Check sheet for the modelled part. Datum: model origin and axes. Units: mm. Coordinates: 2 decimals unless noted, no trailing zeros. Loops run counter-clockwise (first coordinate to the right, second up) from the corner with the lowest first, then second, coordinate; pieces in that order, holes last. Notation, with made-up numbers: M -3,62.5 L 55,62.5 A12 cw 55,77.5 Z; hole C -22,59 d4. An arc over 180 degrees is marked long. Answer as CSV lines item,"result". Start each with the question number.
Autodesk Inventor part; units mm, degrees
ref_plane "Work Plane1" through (0, 0, 20) normal (1, 0, 0) x (0, 0, -1)
ref_plane "Work Plane2" through (-25, 0, 0) normal (0, 0, 1) x (1, 0, 0)
ref_plane "YZ Plane" through (0, 0, 0) normal (1, 0, 0) x (0, 1, 0)
sketch "Sketch1" plane through (0, 0, 0) normal (0, 1, 0) x (-1, 0, 0)
  circle A0 centre (0, 0) radius 6.5
  line L0 (25, 20) -> (-25, 20)
  line L1 (-25, 20) -> (-25, -20)
  line L2 (-25, -20) -> (25, -20)
  line L3 (25, -20) -> (25, 20)
  line L4 (25, 20) -> (-25, -20) construction
  line L5 (-25, 20) -> (25, -20) construction
  line L6 (-25, 0) -> (-30, 0)
  line L7 (-30, 0) -> (-30, -10)
  line L8 (-30, -10) -> (-25, -10)
  line L9 (-25, -10) -> (-25, 0)
  line L10 (-30, 0) -> (-25, 0)
  line L11 (-25, 0) -> (-25, 10)
  line L12 (-25, 10) -> (-30, 10)
  line L13 (-30, 10) -> (-30, 0)
  line L14 (-25, 10) -> (-25, 5)
  line L15 (-25, 5) -> (-26.5, 5)
  line L16 (-26.5, 5) -> (-28, 5)
  line L17 (-28, 5) -> (-28, -5)
  line L18 (-28, -5) -> (-26.5, -5)
  line L19 (-26.5, -5) -> (-26.5, 5)
  line L20 (0, 0) -> (0, -20)
  line L21 (30, 0) -> (30, -10)
  line L22 (30, -10) -> (25, -10)
  line L23 (26.5, -5) -> (26.5, 5)
  line L24 (28, 5) -> (28, -5)
  line L25 (28, -5) -> (26.5, -5)
  line L26 (26.5, 5) -> (28, 5)
  line L27 (25, 10) -> (30, 10)
  line L28 (30, 10) -> (30, 0)
  dimension "d0" = 13
  dimension "d1" = 50
  dimension "d2" = 40
  dimension "d3" = 5
  dimension "d4" = 10
  dimension "d5" = 5
  dimension "d6" = 10
  dimension "d7" = 5
  dimension "d8" = 1.5
  dimension "d9" = 1.5
  dimension "d10" = 10
extrude "Extrusion1" add sketch "Sketch1" along normal blind 1.5 contours L2 L1 L0 L3 | L8 L7 L6 L17 L18 L19 L1 | L3 L27 L28 L21 L22 | L6 L19 L15 L1 | L15 L16 L17 L6 L13 L12 L1
sketch "Sketch2" plane through (0, 1.5, 0) normal (0, 1, 0) x (1, 0, 0)
  line L0 (0, 0) -> (22.5, 0)
  line L1 (22.5, 0) -> (22.5, 17.5)
  line L2 (25, 20) -> (-25, 20)
  circle A0 centre (22.5, 17.5) radius 1.5
  dimension "d13" = 22.5
  dimension "d14" = 17.5
  dimension "d15" = 3
extrude "Extrusion2" cut sketch "Sketch2" against normal blind 1.5
ref_plane "Work Plane1" through (0, 0, 20) normal (1, 0, 0) x (0, 0, -1)
ref_plane "Work Plane2" through (-25, 0, 0) normal (0, 0, 1) x (1, 0, 0)
mirror "Mirror1" about plane through (0, 0, 20) normal (1, 0, 0) of "Extrusion2"
mirror "Mirror2" about plane through (-25, 0, 0) normal (0, 0, 1) of "Extrusion2", "Mirror1"
sketch "Sketch3" plane through (0, 1.5, 0) normal (0, 1, 0) x (1, 0, 0)
  line L0 (25, 10) -> (25, 20)
  line L1 (25, 20) -> (20, 20)
  line L2 (25, 20) -> (-25, 20)
  line L3 (0, 0) -> (0, 9)
  line L4 (20, 20) -> (9.6256, 9) construction
  line L5 (9.6256, 9) -> (0, 9) construction
  spline S0 degree 2 poles (20, 20) (9.6256, 9) (0, 9) knots 1 1 1 2 2 2
  line L6 (0, 0) -> (9.6256, 0)
  line L7 (-20, 20) -> (-9.6256, 9) construction
  line L8 (-9.6256, 9) -> (0, 9) construction
  spline S1 degree 2 poles (-20, 20) (-9.6256, 9) (0, 9) knots 1 1 1 2 2 2
  line L9 (20, -20) -> (9.6256, -9) construction
  line L10 (9.6256, -9) -> (0, -9) construction
  spline S2 degree 2 poles (20, -20) (9.6256, -9) (0, -9) knots 1 1 1 2 2 2
  line L11 (-20, -20) -> (-9.6256, -9) construction
  spline S3 degree 2 poles (-20, -20) (-9.6256, -9) (0, -9) knots 1 1 1 2 2 2
  line L12 (-9.6256, -9) -> (0, -9) construction
  line L13 (20, 20) -> (-20, 20)
  line L14 (20, -20) -> (-20, -20)
  line L15 (-25, -20) -> (25, -20)
  dimension "d18" = 5
  dimension "d19" = 9
extrude "Extrusion3" cut sketch "Sketch3" against normal blind 1.5
properties part number "bottomBearingHolder"
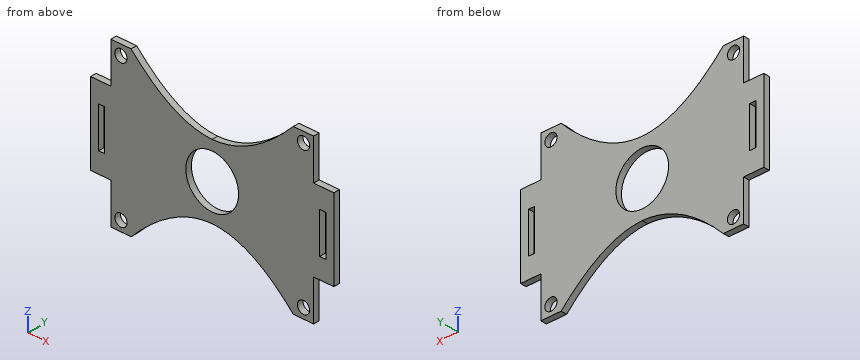
Item 1: Material ranges on line 1 (Z direction, x = 22.5, y = 0.35); line 2 (X direction, y = 0.75, z = 0); line 3 (Z direction, x = 0, y = 0.8), recorded low to high. Write a range as from..to.
Item 2: Sectioned sample at B-B, the plane z = 0. Record the boundary of the cut face in (x, y), and give its area (3 significant figures).
Item 3: Go/stop test with flat-tipped pins: pin 1 (0.8 mm diameter, centred on x = 27.5, y = 0.5, fed in from +Z); pin 2 (0.8 mm diameter, centred on y = 0.5, z = 12.5, fed in from -X). Record where each tip stops, or that it passes through.
Item 4: Sectioned sample at A-A, the plane x = -22.5. Record the boundary of the cut face in (y, z).
Item 5: Sectioned sample at C-C, the plane y = 1.15. Give the number of separate pieces and of enclosed holes in the cut face, and give its area (3 significant figures).
Reply:
1,line 1,"-20..-19, -16..16, 19..20"
1,line 2,"-30..-28, -26.5..-6.5, 6.5..26.5, 28..30"
1,line 3,"-9..-6.5, 6.5..9"
2,outline,"M -30,0 L -28,0 L -28,1.5 L -30,1.5 Z; M -26.5,0 L -6.5,0 L -6.5,1.5 L -26.5,1.5 Z; M 6.5,0 L 26.5,0 L 26.5,1.5 L 6.5,1.5 Z; M 28,0 L 30,0 L 30,1.5 L 28,1.5 Z"
2,area,"66.0 mm²"
3,pin 1,"z = 10"
3,pin 2,"x = -25"
4,outline,"M 0,-20 L 1.5,-20 L 1.5,-19 L 0,-19 Z; M 0,-16 L 1.5,-16 L 1.5,16 L 0,16 Z; M 0,19 L 1.5,19 L 1.5,20 L 0,20 Z"
5,separate pieces,"1"
5,enclosed holes,"7"
5,area,"1,430 mm²"
